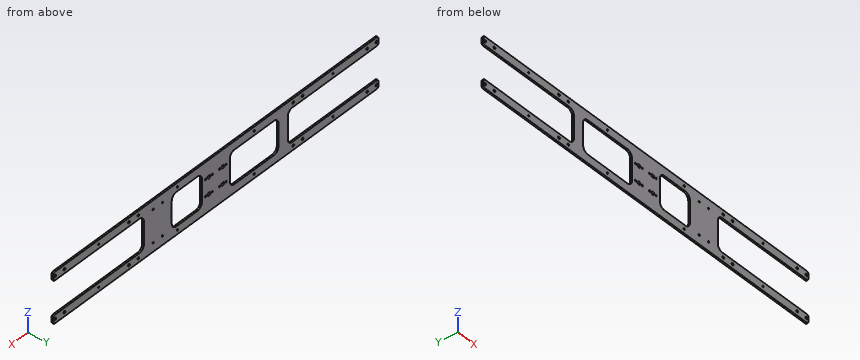
from build123d import *

# Parameters (mm, degrees)
SKETCH_1_W                                   = 700
SKETCH_1_H                                   = 90
SKETCH_1_W_2                                 = 270
SKETCH_1_H_2                                 = 60
EXTRUDE_1_DEPTH                              = 3
SKETCH_2_W                                   = 195
SKETCH_2_H                                   = 60
CUT_EXTRUDE_1_DEPTH                          = 4
SKETCH_4_R                                   = 2
CUT_EXTRUDE_2_DEPTH                          = 15
MIRROR_2_AT_THE_SECOND_PLANE_COPY_1_SKET_R   = 2
MIRROR_2_AT_THE_SECOND_PLANE_COPY_1_DEPTH    = 15
SKETCH_5_W                                   = 60
SKETCH_5_H                                   = 60
EXTRUDE_2_DEPTH                              = 3
SKETCH_6_R                                   = 1.5
CUT_EXTRUDE_3_DEPTH                          = 4
MIRROR_3_AT_THE_SECOND_PLANE_COPY_1_SKET_R   = 1.5
MIRROR_3_AT_THE_SECOND_PLANE_COPY_1_DEPTH    = 4
SKETCH_9_W                                   = 40
SKETCH_9_H                                   = 60
EXTRUDE_4_DEPTH                              = 3
FILLET_1_R                                   = 2
MIRROR_6_DEPTH                               = 3
EXTRUDE_3_DEPTH                              = 3
MIRROR_9_AT_THE_SECOND_PLANE_COPY_1_DEPTH    = 3
SKETCH_8_R                                   = 3
SKETCH_8_R_2                                 = 1.5
CUT_EXTRUDE_4_DEPTH                          = 15
SKETCH_10_R                                  = 1.5
CUT_EXTRUDE_5_DEPTH                          = 38
MIRROR_10_AT_THE_SECOND_PLANE_COPY_1_SKE_R   = 3
MIRROR_10_AT_THE_SECOND_PLANE_COPY_1_SKE_R_2 = 1.5
MIRROR_10_AT_THE_SECOND_PLANE_COPY_1_DEPTH   = 15
FILLET_2_R                                   = 10


# Read off the part's stored shape, not the designer's step: 镜向6
with BuildPart() as part:
    # 草图1 → 凸台-拉伸1 (new body)
    with BuildSketch(Plane(origin=(0, 0, 0), x_dir=(1, 0, 0), z_dir=(0, 1, 0))):
        Rectangle(SKETCH_1_W, SKETCH_1_H)
        Rectangle(SKETCH_1_W_2, SKETCH_1_H_2, mode=Mode.SUBTRACT)
    extrude(amount=EXTRUDE_1_DEPTH)

    # 草图2 → 切除-拉伸1 (cut)
    with BuildSketch(Plane(origin=(0, 3, 0), x_dir=(1, 0, 0), z_dir=(0, 1, 0))):
        with Locations((-252.5, 0)):
            Rectangle(SKETCH_2_W, SKETCH_2_H)
    cut_extrude_1 = extrude(amount=-CUT_EXTRUDE_1_DEPTH, mode=Mode.SUBTRACT)

    # 镜向1: 切除-拉伸1 across plane
    add(cut_extrude_1.mirror(Plane(origin=(0, 0, 0), x_dir=(0, 0, 1), z_dir=(1, 0, 0))), mode=Mode.SUBTRACT)

    # 草图4 → 切除-拉伸2 (cut)
    with BuildSketch(Plane(origin=(0, 3, 0), x_dir=(1, 0, 0), z_dir=(0, 1, 0))):
        with Locations(Location((-187, 37.5, 0), (0, 0, 270))):
            Circle(SKETCH_4_R)
        with Locations(Location((-167, 37.5, 0), (0, 0, 270))):
            Circle(SKETCH_4_R)
        with Locations(Location((-346, 37.5, 0), (0, 0, 270))):
            Circle(SKETCH_4_R)
        with Locations(Location((-326, 37.5, 0), (0, 0, 270))):
            Circle(SKETCH_4_R)
    cut_extrude_2 = extrude(amount=-CUT_EXTRUDE_2_DEPTH, mode=Mode.SUBTRACT)

    # 镜向2: 切除-拉伸2 across plane
    add(cut_extrude_2.mirror(Plane(origin=(0, 0, 0), x_dir=(0, 0, 1), z_dir=(1, 0, 0))), mode=Mode.SUBTRACT)

    # 镜向2 at the second plane: 切除-拉伸2 across plane
    add(cut_extrude_2.mirror(Plane.XY), mode=Mode.SUBTRACT)

    # 镜向2 at the second plane copy 1 sket → 镜向2 at the second plane copy 1 (cut)
    with BuildSketch(Plane(origin=(0, 3, 0), x_dir=(-1, 0, 0), z_dir=(0, 1, 0))):
        with Locations(Location((-187, 37.5, 0), (0, 0, 270))):
            Circle(MIRROR_2_AT_THE_SECOND_PLANE_COPY_1_SKET_R)
        with Locations(Location((-167, 37.5, 0), (0, 0, 270))):
            Circle(MIRROR_2_AT_THE_SECOND_PLANE_COPY_1_SKET_R)
        with Locations(Location((-346, 37.5, 0), (0, 0, 270))):
            Circle(MIRROR_2_AT_THE_SECOND_PLANE_COPY_1_SKET_R)
        with Locations(Location((-326, 37.5, 0), (0, 0, 270))):
            Circle(MIRROR_2_AT_THE_SECOND_PLANE_COPY_1_SKET_R)
    extrude(amount=-MIRROR_2_AT_THE_SECOND_PLANE_COPY_1_DEPTH, mode=Mode.SUBTRACT)

    # 草图5 → 凸台-拉伸2 (add)
    with BuildSketch(Plane(origin=(0, 3, 0), x_dir=(1, 0, 0), z_dir=(0, 1, 0))):
        Rectangle(SKETCH_5_W, SKETCH_5_H)
    extrude(amount=-EXTRUDE_2_DEPTH)

    # 草图6 → 切除-拉伸3 (cut)
    with BuildSketch(Plane(origin=(0, 3, 0), x_dir=(1, 0, 0), z_dir=(0, 1, 0))):
        with Locations(Location((-252.5, 37.5, 0), (0, 0, 270))):
            Circle(SKETCH_6_R)
        with Locations(Location((-82.5, 37.5, 0), (0, 0, 270))):
            Circle(SKETCH_6_R)
    cut_extrude_3 = extrude(amount=-CUT_EXTRUDE_3_DEPTH, mode=Mode.SUBTRACT)

    # 镜向3: 切除-拉伸3 across plane
    add(cut_extrude_3.mirror(Plane.XY), mode=Mode.SUBTRACT)

    # 镜向3 at the second plane: 切除-拉伸3 across plane
    add(cut_extrude_3.mirror(Plane(origin=(0, 0, 0), x_dir=(0, 0, 1), z_dir=(1, 0, 0))), mode=Mode.SUBTRACT)

    # 镜向3 at the second plane copy 1 sket → 镜向3 at the second plane copy 1 (cut)
    with BuildSketch(Plane(origin=(0, 3, 0), x_dir=(-1, 0, 0), z_dir=(0, 1, 0))):
        with Locations(Location((-252.5, 37.5, 0), (0, 0, 270))):
            Circle(MIRROR_3_AT_THE_SECOND_PLANE_COPY_1_SKET_R)
        with Locations(Location((-82.5, 37.5, 0), (0, 0, 270))):
            Circle(MIRROR_3_AT_THE_SECOND_PLANE_COPY_1_SKET_R)
    extrude(amount=-MIRROR_3_AT_THE_SECOND_PLANE_COPY_1_DEPTH, mode=Mode.SUBTRACT)

    # 草图9 → 凸台-拉伸4 (add)
    with BuildSketch(Plane(origin=(0, 3, 0), x_dir=(1, 0, 0), z_dir=(0, 1, 0))):
        with Locations((115, 0)):
            Rectangle(SKETCH_9_W, SKETCH_9_H)
    extrude(amount=-EXTRUDE_4_DEPTH)

    # 圆角1
    fillet_1_edges = [part.edges().sort_by_distance(p)[0] for p in [
        (-350, 1.5, -30),
        (-350, 1.5, -45),
    ]]
    fillet(fillet_1_edges, radius=FILLET_1_R)

    # 镜向6 outline → 镜向6 (cut)
    with BuildSketch(Plane(origin=(0, 0, 0), x_dir=(1, 0, 0), z_dir=(0, 1, 0))):
        with BuildLine():
            Line((350, 45), (348, 45))
            ThreePointArc((348, 45), (349.414213562, 44.414213562), (350, 43))
            Line((350, 43), (350, 45))
        make_face()
        with BuildLine():
            Line((350, 30), (350, 32))
            ThreePointArc((350, 32), (349.414213562, 30.585786438), (348, 30))
            Line((348, 30), (350, 30))
        make_face()
        with BuildLine():
            Line((-350, -45), (-348, -45))
            ThreePointArc((-348, -45), (-349.414213562, -44.414213562), (-350, -43))
            Line((-350, -43), (-350, -45))
        make_face()
        with BuildLine():
            ThreePointArc((348, -30), (349.414213562, -30.585786438), (350, -32))
            Line((350, -32), (350, -30))
            Line((350, -30), (348, -30))
        make_face()
        with BuildLine():
            ThreePointArc((350, -43), (349.414213562, -44.414213562), (348, -45))
            Line((348, -45), (350, -45))
            Line((350, -45), (350, -43))
        make_face()
        with BuildLine():
            Line((-350, -30), (-350, -32))
            ThreePointArc((-350, -32), (-349.414213562, -30.585786438), (-348, -30))
            Line((-348, -30), (-350, -30))
        make_face()
    extrude(amount=MIRROR_6_DEPTH, mode=Mode.SUBTRACT)

    # 草图7 → 凸台-拉伸3 (add)
    with BuildSketch(Plane(origin=(0, 3, 0), x_dir=(1, 0, 0), z_dir=(0, 1, 0))):
        with BuildLine():
            Line((-165, 30), (-155, 30))
            Line((-155, 30), (-155, 20))
            ThreePointArc((-155, 20), (-157.928932188, 27.071067812), (-165, 30))
        make_face()
        with BuildLine():
            Line((-135, 20), (-135, 30))
            Line((-135, 30), (-125, 30))
            ThreePointArc((-125, 30), (-132.071067812, 27.071067812), (-135, 20))
        make_face()
        with BuildLine():
            Line((-40, 30), (-30, 30))
            Line((-30, 30), (-30, 20))
            ThreePointArc((-30, 20), (-32.928932188, 27.071067812), (-40, 30))
        make_face()
    extrude_3 = extrude(amount=-EXTRUDE_3_DEPTH)

    # 镜向9: 凸台-拉伸3 across plane
    add(extrude_3.mirror(Plane(origin=(0, 0, 0), x_dir=(0, 0, 1), z_dir=(1, 0, 0))))

    # 镜向9 at the second plane: 凸台-拉伸3 across plane
    add(extrude_3.mirror(Plane.XY))

    # 镜向9 at the second plane copy 1 sket → 镜向9 at the second plane copy 1 (add)
    with BuildSketch(Plane(origin=(0, 3, 0), x_dir=(-1, 0, 0), z_dir=(0, 1, 0))):
        with BuildLine():
            Line((-165, 30), (-155, 30))
            Line((-155, 30), (-155, 20))
            ThreePointArc((-155, 20), (-157.928932188, 27.071067812), (-165, 30))
        make_face()
        with BuildLine():
            Line((-135, 20), (-135, 30))
            Line((-135, 30), (-125, 30))
            ThreePointArc((-125, 30), (-132.071067812, 27.071067812), (-135, 20))
        make_face()
        with BuildLine():
            Line((-40, 30), (-30, 30))
            Line((-30, 30), (-30, 20))
            ThreePointArc((-30, 20), (-32.928932188, 27.071067812), (-40, 30))
        make_face()
    extrude(amount=-MIRROR_9_AT_THE_SECOND_PLANE_COPY_1_DEPTH)

    # 草图8 → 切除-拉伸4 (cut)
    with BuildSketch(Plane(origin=(0, 3, 0), x_dir=(1, 0, 0), z_dir=(0, 1, 0))):
        with Locations(Location((-15, 15, 0), (0, 0, 270))):
            Circle(SKETCH_8_R)
        with Locations(Location((-22, 15, 0), (0, 0, 270))):
            Circle(SKETCH_8_R_2)
        with Locations(Location((-8, 15, 0), (0, 0, 270))):
            Circle(SKETCH_8_R_2)
    cut_extrude_4 = extrude(amount=-CUT_EXTRUDE_4_DEPTH, mode=Mode.SUBTRACT)

    # 草图10 → 切除-拉伸5 (cut)
    with BuildSketch(Plane(origin=(0, 3, 0), x_dir=(1, 0, 0), z_dir=(0, 1, 0))):
        with Locations(Location((115, 29, 0), (0, 0, 270))):
            Circle(SKETCH_10_R)
        with Locations(Location((135, 29, 0), (0, 0, 270))):
            Circle(SKETCH_10_R)
        with Locations(Location((135, -29, 0), (0, 0, 270))):
            Circle(SKETCH_10_R)
        with Locations(Location((115, -29, 0), (0, 0, 270))):
            Circle(SKETCH_10_R)
    extrude(amount=-CUT_EXTRUDE_5_DEPTH, mode=Mode.SUBTRACT)

    # 镜向10: 切除-拉伸4 across plane
    add(cut_extrude_4.mirror(Plane.XY), mode=Mode.SUBTRACT)

    # 镜向10 at the second plane: 切除-拉伸4 across plane
    add(cut_extrude_4.mirror(Plane(origin=(0, 0, 0), x_dir=(0, 0, 1), z_dir=(1, 0, 0))), mode=Mode.SUBTRACT)

    # 镜向10 at the second plane copy 1 ske → 镜向10 at the second plane copy 1 (cut)
    with BuildSketch(Plane(origin=(0, 3, 0), x_dir=(-1, 0, 0), z_dir=(0, 1, 0))):
        with Locations(Location((-15, 15, 0), (0, 0, 270))):
            Circle(MIRROR_10_AT_THE_SECOND_PLANE_COPY_1_SKE_R)
        with Locations(Location((-22, 15, 0), (0, 0, 270))):
            Circle(MIRROR_10_AT_THE_SECOND_PLANE_COPY_1_SKE_R_2)
        with Locations(Location((-8, 15, 0), (0, 0, 270))):
            Circle(MIRROR_10_AT_THE_SECOND_PLANE_COPY_1_SKE_R_2)
    extrude(amount=-MIRROR_10_AT_THE_SECOND_PLANE_COPY_1_DEPTH, mode=Mode.SUBTRACT)

    # 圆角2
    fillet_2_edges = [part.edges().sort_by_distance(p)[0] for p in [
        (95, 1.5, -30),
        (95, 1.5, 30),
    ]]
    fillet(fillet_2_edges, radius=FILLET_2_R)


solid = part.part
Geometry: final body of the model. Coordinates: model frame, mm. Coordinates: 2 decimals unless noted, no trailing zeros. Loops run counter-clockwise (first coordinate to the right, second up) from the corner with the lowest first, then second, coordinate; pieces in that order, holes last. Notation, with made-up numbers: M 22.5,34.25 L 42.5,34.25 A20 cw 42.5,63.25 Z; hole C 71,-7.5 d4. An arc over 180 degrees is marked long. One line per item, written item: value. Start each with the question number.
1) Cut plane B-B (y = 0.7). Count the separate pieces of the cut face and the enclosed holes in it, then the cut area to 3 significant figures.
2) Material intervals for L1, parallel to X at y = 2.85, z = -4; L2, parallel to Z at x = 252.5, y = 0.8; L3, parallel to Z at x = 212.5, y = 2.7, sorted ascending. Write a range as from..to.
3) Cut plane A-A (z = 2). Return loops of the section in (x, y).
4) Pin query (flat end, axial travel): P1, Ø0.9, axis at y = 1.5, z = -6, coming from the -X side. Return the tip coordinate at first contact, or that it passes through.
Evaluation:
1. separate pieces: 1
1. enclosed holes: 42
1. area: 29,200 mm^2
2. L1: -155..-135, -30..30, 95..155
2. L2: -45..-39, -36..-30, 30..36, 39..45
2. L3: -45..-30, 30..45
3. outline: M -155,0 L -135,0 L -135,3 L -155,3 Z; M -30,0 L 30,0 L 30,3 L -30,3 Z; M 95,0 L 155,0 L 155,3 L 95,3 Z
4. P1: x = -155
